from build123d import *

# Parameters (mm, degrees)
F0_W      = 84
F0_H      = 70
F0_R      = 16
F1_DEPTH  = 25
F3_D      = 3.2
F3_DEPTH  = 8
F3_TIP    = 0.9613769904
F5_D      = 4.1
F5_DEPTH  = 20
F5_TIP    = 1.231764269
F7_D      = 4.1
F7_DEPTH  = 20
F7_TIP    = 1.231764269
F9_D      = 5
F9_DEPTH  = 20
F9_TIP    = 1.5021515476
F11_D     = 5
F11_DEPTH = 12
F11_TIP   = 1.5021515476
F13_D     = 3.2
F13_DEPTH = 8
F13_TIP   = 0.9613769904


with BuildPart() as f1:
    # F0 (on Front) → F1 (new body)
    with BuildSketch(Plane.XZ):
        Rectangle(F0_W, F0_H)
        with Locations((-18, -5)):
            Circle(F0_R, mode=Mode.SUBTRACT)
    extrude(amount=F1_DEPTH)

    # F3
    with Locations(Plane.XZ.offset(25)):
        with Locations((-36.5, -5), (0.5, -5)):
            Hole(F3_D / 2, depth=F3_DEPTH)
            with Locations((0, 0, -(F3_DEPTH + F3_TIP / 2))):  # 118° drill point
                Cone(0, F3_D / 2, F3_TIP, mode=Mode.SUBTRACT)

    # F5
    with Locations(Plane.XZ.offset(25)):
        with Locations((35, 13), (35, -10), (35, -20)):
            Hole(F5_D / 2, depth=F5_DEPTH)
            with Locations((0, 0, -(F5_DEPTH + F5_TIP / 2))):  # 118° drill point
                Cone(0, F5_D / 2, F5_TIP, mode=Mode.SUBTRACT)

    # F7
    with Locations(Plane.XY.offset(35)):
        with Locations((-18, -12.5)):
            Hole(F7_D / 2, depth=F7_DEPTH)
            with Locations((0, 0, -(F7_DEPTH + F7_TIP / 2))):  # 118° drill point
                Cone(0, F7_D / 2, F7_TIP, mode=Mode.SUBTRACT)

    # F9
    with Locations(Plane.YZ.offset(42)):
        with Locations((-18.5, 24), (-6.5, 24)):
            Hole(F9_D / 2, depth=F9_DEPTH)
            with Locations((0, 0, -(F9_DEPTH + F9_TIP / 2))):  # 118° drill point
                Cone(0, F9_D / 2, F9_TIP, mode=Mode.SUBTRACT)

    # F11
    with Locations(Plane.YZ.offset(42)):
        with Locations((-18.5, 1.5), (-6.5, 1.5)):
            Hole(F11_D / 2, depth=F11_DEPTH)
            with Locations((0, 0, -(F11_DEPTH + F11_TIP / 2))):  # 118° drill point
                Cone(0, F11_D / 2, F11_TIP, mode=Mode.SUBTRACT)

    # F13
    with Locations(Plane(origin=(0, 0, 0), x_dir=(-1, 0, 0), z_dir=(0, 1, 0))):
        with Locations((-0.5, -5), (36.5, -5)):
            Hole(F13_D / 2, depth=F13_DEPTH)
            with Locations((0, 0, -(F13_DEPTH + F13_TIP / 2))):  # 118° drill point
                Cone(0, F13_D / 2, F13_TIP, mode=Mode.SUBTRACT)


solid = f1.part
Could you check a few things on this model? Use its own coordinates, in mm. A direction names the side the tool comes from. Coordinates: 2 decimals unless noted, no trailing zeros. Write each loop counter-clockwise with the first axis right and the second up, starting at its lowest first coordinate (ties: lowest second). Pieces come first, ordered by that corner, then holes. Notation, with made-up numbers: (7, 87) - (35, 87) arc R22 ccw to (35, 112) - close; hole circle Ø9 at (70, 73.5). An arc over 180 degrees is marked (long way). Put each result on its own line as item: value. Start each with the question number.
Q1. I want a section at A-A on z = -13. Write out the boundary of the cut face in (x, y).
Q2. Please list where these lines run through material, in increasing order: L1, parallel to Y at x = 34, z = 1.5; L2, parallel to X at y = -20.75, z = 13; L3, parallel to Z at x = 32, y = -18.5.
Q3. Which directions (+Z, -Z, +X, -X, +Y, -Y) give clear straight access to the entire face, cutting with the end or side of a thin tool? Please do faces 5 (the cylindrical face through (-35.32, -20.94, -3.92)), 6 (the cylindrical face through (32, -8, 26)), 7 (the cylindrical face through (-37.68, -4.06, -3.92)), 8 (the cylindrical face through (-16.373, -13.747, 24.86)).
Q4. Thinking about a two-plate mould opening in Z: for faces 1 (the conical face through (34.74, -3.98, 13.24)), 2 (the flat face through (-1, 0, 0)), 3 (the conical face through (-36.721, -16.206, -5.169)), 4 (the flat face through (-1, -12, 35)), which applies, pulls with the +Z half, pulls with the -Z half, needs draft (parallel to the pull), parting line crosses it, or undercut?
Q5. I'm going to push flat-ended pins straight in: P1, Ø3, axis at y = -6.5, z = 24, coming from the +X side; P2, Ø3, axis at x = 0.5, z = -5, coming from the -Y side; P3, Ø2, axis at x = -23.5, z = -17.5, coming from the -Y side. Where does each tip first touch, or does it pass through?
Checks:
1. outline: (-42, -25) - (-31.86, -25) - (-31.86, 0) - (-42, 0) - close; (-4.14, -25) - (42, -25) - (42, 0) - (-4.14, 0) - close
2. L1: -25 to -21, -16 to -9, -4 to 0
2. L2: -42 to 32.95, 37.05 to 42
2. L3: -35 to -1, 4 to 21.5, 26.5 to 35
3. face 5: -Y
3. face 6: +X
3. face 7: +Y
3. face 8: +Z
4. face 1: undercut
4. face 2: needs draft
4. face 3: undercut
4. face 4: pulls with the +Z half
5. P1: x = 21.4
5. P2: y = -16.94
5. P3: through
